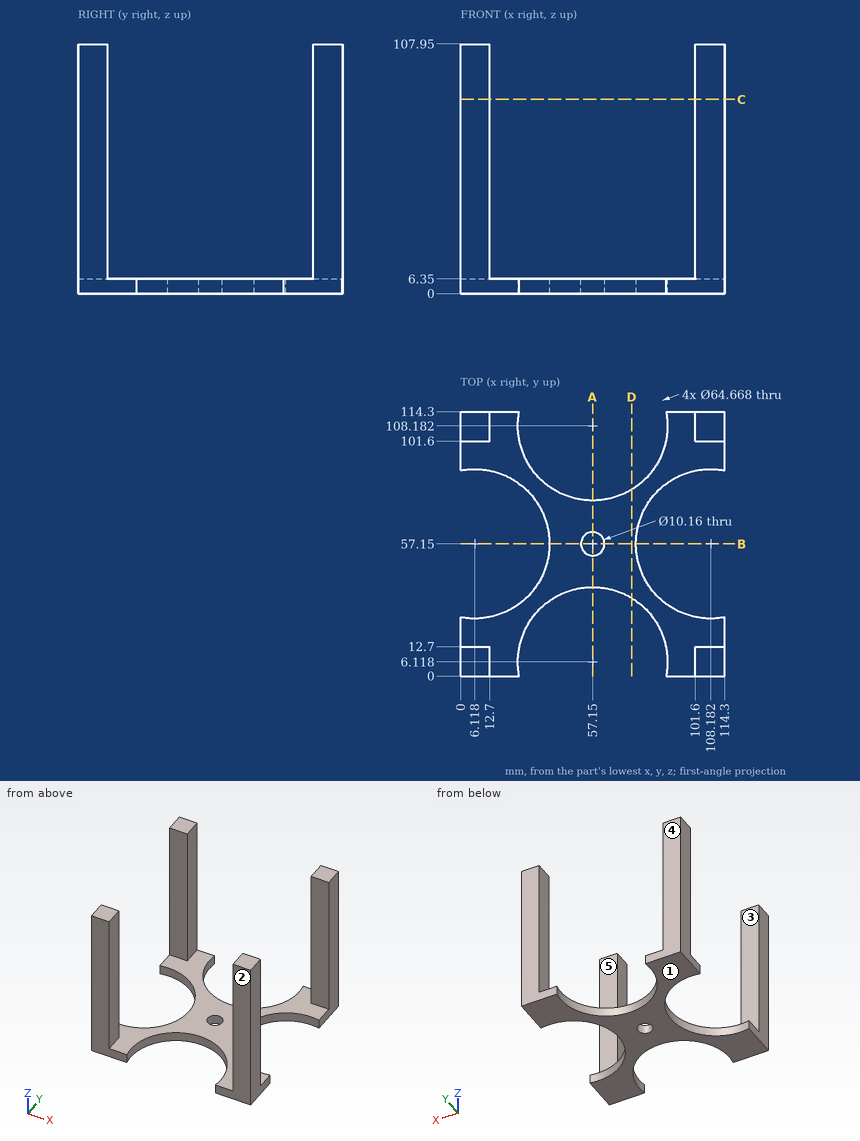
The figure shows three views and two pictorial views of one solid part (mm, origin at its lowest corner). Answer the questions. A direction names the side the tool comes from. Coordinates: 2 decimals unless noted, no trailing zeros. Loops run counter-clockwise (first coordinate to the right, second up) from the corner with the lowest first, then second, coordinate; pieces in that order, holes last. Notation, with made-up numbers: (39, 23.5) - (96, 23.5) arc R20 ccw to (96, 50.5) - close; hole circle Ø9 at (24.25, -15.5). An arc over 180 degrees is marked (long way). Write item = value, one per line.
1) Section D-D (x = 74) is taken. Determine the outline of the cut face in (y, z), plus the area to 3 significant figures.
Responses:
outline = (33.71, 0) - (80.59, 0) - (80.59, 6.35) - (33.71, 6.35) - close
area = 298 mm^2
2) Determine the mould class of the marked faces 1, 2 and 3 for opening direction Y: pulls with the +Y half, pulls with the -Y half, needs draft (parallel to the pull), parting line crosses it, or undercut.
Responses:
face_1 = needs draft
face_2 = pulls with the -Y half
face_3 = undercut
3) Find the intervals of material crossed by line 1 along Y through (x, z) = (12.5, 84.5); line 2 along Y through (x, z) = (57, 2), in increasing order.
Responses:
line_1 = 0 to 12.7, 101.6 to 114.3
line_2 = 38.45 to 52.07, 62.23 to 75.85
4) Section C-C (z = 84) is taken. Determine the outline of the cut face in (x, y), plus the area to 3 significant figures.
Responses:
outline = (0, 0) - (12.7, 0) - (12.7, 12.7) - (0, 12.7) - close; (0, 101.6) - (12.7, 101.6) - (12.7, 114.3) - (0, 114.3) - close; (101.6, 0) - (114.3, 0) - (114.3, 12.7) - (101.6, 12.7) - close; (101.6, 101.6) - (114.3, 101.6) - (114.3, 114.3) - (101.6, 114.3) - close
area = 645 mm^2
5) Which of the six approach directions +Z, -Z, +X, -X, +Y, -Y give full straight-line access (tool end or side, diameter ignored) to the marked faces 4 and 5?
Responses:
face_4 = +Z, -Z, +X, -X, +Y
face_5 = +Z, +X, -X
6) Section A-A (x = 57.15) is taken. Determine the outline of the cut face in (y, z).
Responses:
outline = (38.45, 0) - (52.07, 0) - (52.07, 6.35) - (38.45, 6.35) - close; (62.23, 0) - (75.85, 0) - (75.85, 6.35) - (62.23, 6.35) - close
7) This flat-tipped pin is pushed along its axis until it touches: P1, Ø4, axis at x = 62.5, y = 36.5, coming from the +Z side. Where does it stop, or does it pass through?
Responses:
P1 = 6.35
